Read the model definition and answer for the solid it produces. Units are mm, in the model's axes. Face numbers are marked on the shaded views. A direction names the side the tool comes from. Coordinates: 2 decimals unless noted, no trailing zeros. Order: outer loops, then holes, each group sorted by start corner. A loop starts at its lowest first (then second) coordinate and runs counter-clockwise, first axis right, second up. Notation, with made-up numbers: M -20,65.25 L 19,65.25 A18 cw 19,85.25 Z; hole C 22.5,25 d3. An arc over 180 degrees is marked long. Put each result on its own line as item: value.
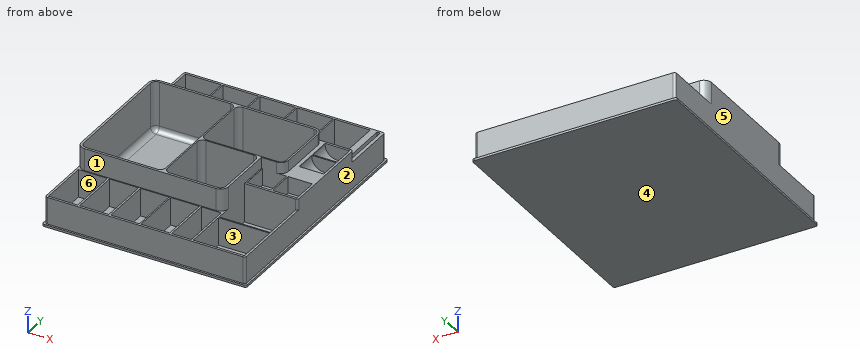
from build123d import *

# Parameters (mm, degrees)
F0_W      = 180
F0_H      = 215
F1_DEPTH  = 25
F2_W      = 166
F2_H      = 46
F2_W_2    = 53
F2_W_3    = 26.2
F2_W_4    = 46
F2_H_2    = 38.8
F2_W_5    = 52.9
F2_H_3    = 55.8
F2_W_6    = 45
F2_H_4    = 24
F2_W_7    = 22
F2_H_5    = 40
F2_W_8    = 73.9
F2_H_6    = 56
F2_H_7    = 113
F2_W_9    = 17.8
F2_W_10   = 3
F3_DEPTH  = 25.001
F4_W      = 180
F4_H      = 215
F5_DEPTH  = 1.2
F6_W      = 1.2
F6_H      = 46
F6_W_2    = 22
F6_H_2    = 1.2
F6_H_3    = 24
F7_DEPTH  = 25
F8_W      = 52.9
F8_H      = 55.8
F8_W_2    = 21.9
F8_H_2    = 24
F8_W_3    = 73.9
F8_H_3    = 113
F8_H_4    = 56
F8_W_4    = 22
F8_H_5    = 19.4
F9_DEPTH  = 20
F10_W     = 24
F10_H     = 20
F11_DEPTH = 45
F13_DEPTH = 40
F14_W     = 183.4
F14_H     = 218.4
F14_W_2   = 180
F14_H_2   = 215
F15_DEPTH = 2
F17_DEPTH = 10
F18_R     = 2
F19_R     = 5
F20_R     = 7


with BuildPart() as f1:
    # F0 (on Top) → F1 (new body)
    with BuildSketch(Plane.XY):
        with Locations((90, 107.5)):
            Rectangle(F0_W, F0_H)
    extrude(amount=F1_DEPTH)

    # F2 (on face) → F3 (cut, through all)
    with BuildSketch(Plane.XY.offset(25)):
        with Locations((85, 190)):
            Rectangle(F2_W, F2_H)
        with Locations((84.3, 25)):
            Rectangle(F2_W_2, F2_H)
        with Locations((15.1, 25)):
            Rectangle(F2_W_3, F2_H)
        with Locations((155, 21.4)):
            Rectangle(F2_W_4, F2_H_2)
        with Locations((155, 61.4)):
            Rectangle(F2_W_4, F2_H_2)
        with Locations((43, 25)):
            Rectangle(F2_W_3, F2_H)
        with Locations((103.55, 78.9)):
            Rectangle(F2_W_5, F2_H_3)
        with Locations((155.5, 94.8)):
            Rectangle(F2_W_6, F2_H_4)
        with Locations((167, 144)):
            Rectangle(F2_W_7, F2_H_5)
        with Locations((114.05, 136)):
            Rectangle(F2_W_8, F2_H_6)
        with Locations((38.95, 107.5)):
            Rectangle(F2_W_8, F2_H_7)
        with Locations((121.4, 25)):
            Rectangle(F2_W_9, F2_H)
        with Locations((175.5, 190)):
            Rectangle(F2_W_10, F2_H)
    extrude(amount=-F3_DEPTH, mode=Mode.SUBTRACT)

    # F4 (on Top) → F5 (join)
    with BuildSketch(Plane.XY):
        with Locations((90, 107.5)):
            Rectangle(F4_W, F4_H)
    extrude(amount=-F5_DEPTH)

    # F6 (on Top) → F7 (join, through all)
    with BuildSketch(Plane.XY):
        with Locations((34.84, 190)):
            Rectangle(F6_W, F6_H)
        with Locations((68.28, 190)):
            Rectangle(F6_W, F6_H)
        with Locations((101.72, 190)):
            Rectangle(F6_W, F6_H)
        with Locations((135.16, 190)):
            Rectangle(F6_W, F6_H)
        with Locations((84.3, 25)):
            Rectangle(F6_W, F6_H)
        with Locations((167, 144)):
            Rectangle(F6_W_2, F6_H_2)
        with Locations((155.5, 94.8)):
            Rectangle(F6_W, F6_H_3)
    extrude(amount=F7_DEPTH)

    # F8 (on face) → F9 (join)
    with BuildSketch(Plane.XY.offset(25)):
        Polygon((0, 166), (0, 49), (132, 49), (132, 80.8), (180, 80.8), (180, 166), (132, 166), align=None)
        with Locations((103.55, 78.9)):
            Rectangle(F8_W, F8_H, mode=Mode.SUBTRACT)
        with Locations((143.95, 94.8)):
            Rectangle(F8_W_2, F8_H_2, mode=Mode.SUBTRACT)
        with Locations((167.05, 94.8)):
            Rectangle(F8_W_2, F8_H_2, mode=Mode.SUBTRACT)
        with Locations((38.95, 107.5)):
            Rectangle(F8_W_3, F8_H_3, mode=Mode.SUBTRACT)
        with Locations((114.05, 136)):
            Rectangle(F8_W_3, F8_H_4, mode=Mode.SUBTRACT)
        with Locations((167, 133.7)):
            Rectangle(F8_W_4, F8_H_5, mode=Mode.SUBTRACT)
        with Locations((167, 154.3)):
            Rectangle(F8_W_4, F8_H_5, mode=Mode.SUBTRACT)
    extrude(amount=F9_DEPTH)

    # F10 (on face) → F11 (join, through all)
    with BuildSketch(Plane.YZ.offset(133)):
        with Locations((94.8, 10)):
            Rectangle(F10_W, F10_H)
    extrude(amount=F11_DEPTH)

    # F12 (on face) → F13 (join, through all)
    with BuildSketch(Plane.XZ.offset(-164)):
        with BuildLine():
            Line((156, 34), (156, 0))
            Line((156, 0), (178, 0))
            Line((178, 0), (178, 34))
            ThreePointArc((178, 34), (167, 23), (156, 34))
        make_face()
    extrude(amount=F13_DEPTH)

    # F14 (on face) → F15 (join)
    with BuildSketch(Plane(origin=(0, 0, -1.2), x_dir=(1, 0, 0), z_dir=(0, 0, -1))):
        with Locations((90, -107.5)):
            Rectangle(F14_W, F14_H)
        with Locations((90, -107.5)):
            Rectangle(F14_W_2, F14_H_2, mode=Mode.SUBTRACT)
    extrude(amount=-F15_DEPTH)

    # F16 (on face) → F17 (cut)
    with BuildSketch(Plane.XY.offset(45)):
        Polygon((132, 106.8), (132, 80.8), (180, 80.8), (180, 166), (152.5, 166), (152.5, 106.8), align=None)
    extrude(amount=-F17_DEPTH, mode=Mode.SUBTRACT)

    # F18
    f18_edges = [f1.edges().sort_by_distance(p)[0] for p in [
        (180, 0, 12.9),
        (180, 80.8, 30),
        (180, 166, 30),
        (180, 215, 12.9),
        (0, 215, 12.9),
        (0, 0, 12.9),
        (-1.7, -1.7, -0.2),
        (181.7, -1.7, -0.2),
        (181.7, 216.7, -0.2),
        (-1.7, 216.7, -0.2),
    ]]
    fillet(f18_edges, radius=F18_R)

    # F19
    f19_edges = [f1.edges().sort_by_distance(p)[0] for p in [
        (77.1, 78.9, 0),
        (103.55, 106.8, 0),
        (130, 78.9, 0),
        (103.55, 51, 0),
        (77.1, 136, 0),
        (114.05, 164, 0),
        (151, 136, 0),
        (114.05, 108, 0),
        (38.95, 164, 0),
        (75.9, 107.5, 0),
        (38.95, 51, 0),
        (2, 107.5, 0),
        (2, 51, 22.5),
        (2, 164, 22.5),
        (75.9, 164, 22.5),
        (75.9, 51, 22.5),
        (77.1, 106.8, 22.5),
        (77.1, 164, 22.5),
        (151, 164, 22.5),
        (151, 108, 22.5),
        (130, 106.8, 22.5),
        (130, 51, 22.5),
        (77.1, 51, 22.5),
        (77.1, 108, 22.5),
    ]]
    fillet(f19_edges, radius=F19_R)

    # F20
    f20_edges = [f1.edges().sort_by_distance(p)[0] for p in [
        (132, 49, 35),
        (0, 49, 35),
        (152.5, 106.8, 40),
        (152.5, 166, 40),
        (0, 166, 35),
    ]]
    fillet(f20_edges, radius=F20_R)


solid = f1.part
Q1. Given pin 1 (16 mm diameter, centred on x = 80, y = 192, fed in from +Z); pin 2 (20 mm diameter, centred on x = 155, z = 11.5, fed in from +Y); pin 3 (6 mm diameter, centred on y = 84, z = 10, fed in from -X), each flat-ended and moving along its own axis, determine where each tip first touches the part or whether it passes through.
Answers below:
pin 1: stops at z = 0
pin 2: stops at y = 215
pin 3: stops at x = 0
Q2. A tool of negligible diameter and unlimited length cuts with its end or side. For the marked faces 4, 5 and 6, from which of +Z, -Z, +X, -X, +Y, -Y can it reach the whole face along a straight path? Write none if from no direction.
Answers below:
face 4: -Z, +X, -X, +Y, -Y
face 5: +Z, -X, +Y, -Y
face 6: +Z
Q3. Consider line 1 along X through (y, z) = (88, 8.5); line 2 along Y through (x, z) = (153, 18); line 3 along Y through (x, z) = (101.5, 19.5). Determine where each line is inside the solid, lowest interval first.
Answers below:
line 1: x = 0 to 2, 75.9 to 77.1, 130 to 180
line 2: y = 0 to 2, 40.8 to 42, 80.8 to 167, 213 to 215
line 3: y = 0 to 2, 48 to 51, 106.8 to 108, 164 to 215
Q4. Find section C-C on z = 17.5. Give the number of separate pieces and of enclosed holes in the cut face, plus the area to 3 significant figures.
Answers below:
separate pieces: 1
enclosed holes: 16
area: 6,590 mm^2
Q5. Find section D-D on y = 67. Write down the section's boundary in (x, z).
Answers below:
outline: M -1.7,-1.2 L 181.7,-1.2 L 181.7,0.8 L 180,0.8 L 180,25 L 178,25 L 178,0 L 132,0 L 132,45 L 130,45 L 130,5 A5 cw 125,0 L 82.1,0 A5 cw 77.1,5 L 77.1,45 L 75.9,45 L 75.9,5 A5 cw 70.9,0 L 7,0 A5 cw 2,5 L 2,45 L 0,45 L 0,0.8 L -1.7,0.8 Z
Q6. For a pull along Y with two mould halves and no side action, classify the marked faces 1, 2 and 3 as +Y half, -Y half, draft (parallel to the pull), parting line (faces both ways), or undercut.
Answers below:
face 1: -Y half
face 2: draft
face 3: undercut
